The listing builds one solid part. Answer for the finished solid, in the listing's coordinates (mm). Face numbers are marked on the shaded views. A direction names the side the tool comes from. Round coordinates to 2 decimals unless told otherwise and drop trailing zeros. Order: outer loops, then holes, each group sorted by start corner. A loop starts at its lowest first (then second) coordinate and runs counter-clockwise, first axis right, second up. Notation, with made-up numbers: (87.25, -32.5) - (122.25, -32.5) arc R11 cw to (122.25, -16.5) - close; hole circle Ø2 at (26.25, 2.25). An arc over 180 degrees is marked (long way). Use CSV: the item, a comma, the result in double quotes. Start each with the question number.
Item 1: Determine the mould class of the marked faces 3 and 4 for opening direction Y: +Y half, -Y half, draft (parallel to the pull), parting line (faces both ways), or undercut.
Item 2: Find section B-B, the plane x = 15. Give the vertices of the cut face in (y, z), plus the area to 3 significant figures.
Item 3: Find section A-A, the plane y = -12.25. Give the vertices of the cut face in (x, z), plus the area to 3 significant figures.
Item 4: Find section C-C, the plane z = -94. Give the vertices of the cut face in (x, y).
Item 5: Flat-ended cylindrical pins translate along their axes: P1, Ø11, axis at x = 16.5, z = -133, coming from the +Y side; P2, Ø0.6, axis at y = -29, z = -222.5, coming from the -X side; P3, Ø1.6, axis at y = -28.5, z = -138.5, coming from the +X side; P4, Ø2, axis at y = -0.5, z = -139, coming from the -X side. Find the tip coordinate at first contact, or state that the pin passes through.
Item 6: For the marked faces 1 and 2, determine the directions among +Z, -Z, +X, -X, +Y, -Y from which every point of the face is accessible in a straight line to the end or side of a thin tool.
Item 7: Straight lines are drawn through the part: line 1 along X through (y, z) = (-3.75, -126); line 2 along Y through (x, z) = (23, -13.5); line 3 along Y through (x, z) = (9, -135.5). For each, find the intervals that lie inside material, in ascending order. Write a range as [from, to].
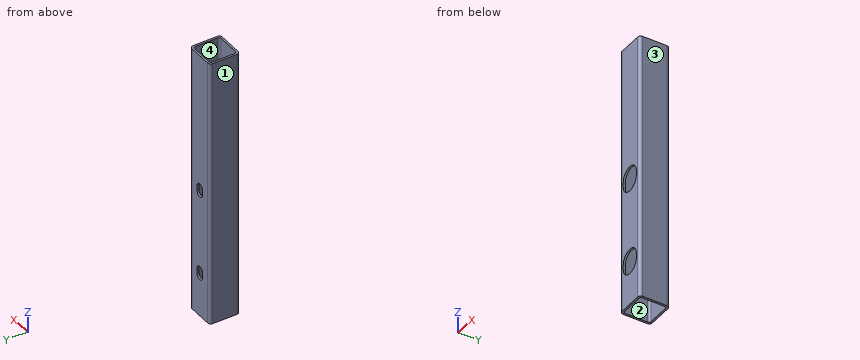
```python
from build123d import *

# Parameters (mm, degrees)
EXTRUDE_1_DEPTH     = 267.336309
CUT_EXTRUDE_1_DEPTH = 31
CUT_EXTRUDE_2_DEPTH = 10


with BuildPart() as part:
    # Эскиз1 → Бобышка-Вытянуть1 (new body)
    with BuildSketch(Plane.XY):
        with BuildLine():
            Line((3, 0), (27, 0))
            ThreePointArc((27, 0), (29.121320344, -0.878679656), (30, -3))
            Line((30, -3), (30, -27))
            ThreePointArc((30, -27), (29.121320344, -29.121320344), (27, -30))
            Line((27, -30), (3, -30))
            ThreePointArc((3, -30), (0.878679656, -29.121320344), (0, -27))
            Line((0, -27), (0, -3))
            ThreePointArc((0, -3), (0.878679656, -0.878679656), (3, 0))
        make_face()
        with BuildLine():
            Line((4, -2), (26, -2))
            ThreePointArc((26, -2), (27.414213562, -2.585786438), (28, -4))
            Line((28, -4), (28, -26))
            ThreePointArc((28, -26), (27.414213562, -27.414213562), (26, -28))
            Line((26, -28), (4, -28))
            ThreePointArc((4, -28), (2.585786438, -27.414213562), (2, -26))
            Line((2, -26), (2, -4))
            ThreePointArc((2, -4), (2.585786438, -2.585786438), (4, -2))
        make_face(mode=Mode.SUBTRACT)
    extrude(amount=-EXTRUDE_1_DEPTH)

    # Эскиз2 → Вырез-Вытянуть1 (cut, through all)
    with BuildSketch(Plane.XZ.offset(30)):
        with BuildLine():
            Line((19.25, -135.836309448), (19.25, -140.836309448))
            ThreePointArc((19.25, -140.836309448), (15, -145.086309448), (10.75, -140.836309448))
            Line((10.75, -140.836309448), (10.75, -135.836309448))
            ThreePointArc((10.75, -135.836309448), (15, -131.586309448), (19.25, -135.836309448))
        make_face()
        with BuildLine():
            Line((10.75, -225.836309448), (10.75, -220.836309448))
            ThreePointArc((10.75, -220.836309448), (15, -216.586309448), (19.25, -220.836309448))
            Line((19.25, -220.836309448), (19.25, -225.836309448))
            ThreePointArc((19.25, -225.836309448), (15, -230.086309448), (10.75, -225.836309448))
        make_face()
    extrude(amount=-CUT_EXTRUDE_1_DEPTH, mode=Mode.SUBTRACT)

    # Эскиз3 → Вырез-Вытянуть2 (cut)
    with BuildSketch(Plane.XZ.offset(30)):
        with BuildLine():
            Line((5, -140.836309448), (5, -135.836309448))
            ThreePointArc((5, -135.836309448), (15, -125.836309448), (25, -135.836309448))
            Line((25, -135.836309448), (25, -140.836309448))
            ThreePointArc((25, -140.836309448), (15, -150.836309448), (5, -140.836309448))
        make_face()
        with BuildLine():
            Line((5, -225.836309448), (5, -220.836309448))
            ThreePointArc((5, -220.836309448), (15, -210.836309448), (25, -220.836309448))
            Line((25, -220.836309448), (25, -225.836309448))
            ThreePointArc((25, -225.836309448), (15, -235.836309448), (5, -225.836309448))
        make_face()
    extrude(amount=-CUT_EXTRUDE_2_DEPTH, mode=Mode.SUBTRACT)


solid = part.part
```
Worked out:
1,face 3,"draft"
1,face 4,"undercut"
2,outline,"(-30, -267.34) - (-28, -267.34) - (-28, -235.84) - (-30, -235.84) - close; (-30, -210.84) - (-28, -210.84) - (-28, -150.84) - (-30, -150.84) - close; (-30, -125.84) - (-28, -125.84) - (-28, 0) - (-30, 0) - close; (-2, -267.34) - (0, -267.34) - (0, -230.09) - (-2, -230.09) - close; (-2, -216.59) - (0, -216.59) - (0, -145.09) - (-2, -145.09) - close; (-2, -131.59) - (0, -131.59) - (0, 0) - (-2, 0) - close"
2,area,"915 mm²"
3,outline,"(0, -267.34) - (2, -267.34) - (2, 0) - (0, 0) - close; (28, -267.34) - (30, -267.34) - (30, 0) - (28, 0) - close"
3,area,"1,070 mm²"
4,outline,"(0, -27) arc R3 ccw to (3, -30) - (27, -30) arc R3 ccw to (30, -27) - (30, -3) arc R3 ccw to (27, 0) - (3, 0) arc R3 ccw to (0, -3) - close; hole (2, -26) arc R2 ccw to (4, -28) - (26, -28) arc R2 ccw to (28, -26) - (28, -4) arc R2 ccw to (26, -2) - (4, -2) arc R2 ccw to (2, -4) - close"
5,P1,"stops at y = 0"
5,P2,"stops at x = 0.53"
5,P3,"stops at x = 29.92"
5,P4,"stops at x = 0.4"
6,face 1,"+Z, -Z, -X, +Y, -Y"
6,face 2,"+Z, -Z"
7,line 1,"x = [0, 2.02], [27.98, 30]"
7,line 2,"y = [-30, -28], [-2, 0]"
7,line 3,"y = [-2, 0]"
